Design review of the part built by this model. Coordinates are the model's own, in mm. A direction names the side the tool comes from. Round coordinates to 2 decimals unless told otherwise and drop trailing zeros. Order: outer loops, then holes, each group sorted by start corner. A loop starts at its lowest first (then second) coordinate and runs counter-clockwise, first axis right, second up.
Autodesk Inventor part; units mm, degrees
ref_plane "YZ Plane" through (0, 0, 0) normal (1, 0, 0) x (0, 1, 0)
ref_plane "XZ Plane" through (0, 0, 0) normal (0, 1, 0) x (-1, 0, 0)
ref_plane "XY Plane" through (0, 0, 0) normal (0, 0, 1) x (1, 0, 0)
sketch "Sketch1" plane through (0, 0, 0) normal (0, 0, 1) x (1, 0, 0)
  line L0 (19.05, -19.05) -> (-19.05, -19.05)
  line L1 (-19.05, -19.05) -> (-19.05, 19.05)
  line L2 (-19.05, 19.05) -> (19.05, 19.05)
  line L3 (19.05, 19.05) -> (19.05, -19.05)
  line L4 (19.05, -19.05) -> (-19.05, 19.05) construction
  line L5 (-19.05, -19.05) -> (19.05, 19.05) construction
  line L6 (-19.05, 19.05) -> (19.05, 19.05)
  line L7 (19.05, 19.05) -> (19.05, 44.45)
  line L8 (19.05, 44.45) -> (-19.05, 44.45)
  line L9 (-19.05, 44.45) -> (-19.05, 19.05)
  line L10 (0, 19.05) -> (0, 82.55)
  circle A0 centre (0, 82.55) radius 47.625
  circle A1 centre (0, 82.55) radius 28.575
  point P0 (0, 0)
  dimension "d0" = 38.1
  dimension "d1" = 38.1
  dimension "d2" = 25.4
  dimension "d3" = 63.5
  dimension "d4" = 95.25
  dimension "d5" = 57.15
extrude "Extrusion1" add sketch "Sketch1" along normal blind 3.175
sketch "Sketch2" plane through (0, 0, 3.175) normal (0, 0, 1) x (1, 0, 0)
  circle A0 centre (0, 82.55) radius 28.575 construction
  arc A1 (19.05, 38.901) -> (-19.05, 38.901) centre (0, 82.55) ccw construction
  line L0 (-19.05, 38.901) -> (-19.05, -19.05) construction
  line L1 (-19.05, -19.05) -> (19.05, -19.05) construction
  line L2 (19.05, -19.05) -> (19.05, 38.901) construction
  line L3 (-19.05, -19.05) -> (19.05, -19.05) construction
  line L4 (19.05, -19.05) -> (19.05, 19.05) construction
  line L5 (19.05, 19.05) -> (-19.05, 19.05) construction
  line L6 (-19.05, 19.05) -> (-19.05, -19.05) construction
  line L7 (15.875, -11.43) -> (-15.875, -11.43) construction
  line L8 (-15.875, -11.43) -> (-15.875, 11.43) construction
  line L9 (-15.875, 11.43) -> (15.875, 11.43) construction
  line L10 (15.875, 11.43) -> (15.875, -11.43) construction
  line L11 (15.875, -11.43) -> (-15.875, 11.43) construction
  line L12 (-15.875, -11.43) -> (15.875, 11.43) construction
  line L13 (11.43, -15.875) -> (-11.43, -15.875) construction
  line L14 (-11.43, -15.875) -> (-11.43, 15.875) construction
  line L15 (-11.43, 15.875) -> (11.43, 15.875) construction
  line L16 (11.43, 15.875) -> (11.43, -15.875) construction
  line L17 (11.43, -15.875) -> (-11.43, 15.875) construction
  line L18 (-11.43, -15.875) -> (11.43, 15.875) construction
  line L19 (0, -8.4414) -> (8.4414, 0) construction
  line L20 (8.4414, 0) -> (0, 8.4414) construction
  line L21 (0, 8.4414) -> (-8.4414, 0) construction
  line L22 (-8.4414, 0) -> (0, -8.4414) construction
  line L23 (-5.969, -5.969) -> (5.969, 5.969) construction
  line L24 (5.969, -5.969) -> (-5.969, 5.969) construction
  line L25 (-8.4414, -8.4414) -> (8.4414, -8.4414) construction
  line L26 (8.4414, -8.4414) -> (8.4414, 8.4414) construction
  line L27 (8.4414, 8.4414) -> (-8.4414, 8.4414) construction
  line L28 (-8.4414, 8.4414) -> (-8.4414, -8.4414) construction
  line L29 (-8.4414, -8.4414) -> (8.4414, 8.4414) construction
  line L30 (8.4414, -8.4414) -> (-8.4414, 8.4414) construction
  point P0 (0, 0)
  point P1 (0, 8.4414)
  point P2 (8.4414, 0)
  point P3 (-15.875, 0)
  point P4 (15.875, 0)
  dimension "d8" = 38.1
  dimension "d9" = 38.1
  dimension "d10" = 31.75
  dimension "d11" = 22.86
  dimension "d12" = 22.86
  dimension "d13" = 31.75
  dimension "d14" = 11.938
  dimension "d15" = 11.938
  dimension "d16" = 16.8829
  dimension "d17" = 16.8829
  dimension "d18" = 4.445
  dimension "d19" = 7.4336
  dimension "d20" = 5.969
  dimension "d21" = 5.969
  dimension "d22" = 4.445
  dimension "d23" = 7.4336
  dimension "d24" = 9.906
  dimension "d25" = 9.906
  dimension "d26" = 21.844
  dimension "d27" = 21.844
  dimension "d28" = 3.175
  dimension "d29" = 27.4914
hole "Hole1" at (-15.875, 11.43, 3.175) at (-15.875, 0, 3.175) at (-15.875, -11.43, 3.175) at (15.875, -11.43, 3.175) at (15.875, 0, 3.175) at (15.875, 11.43, 3.175) at (0, 8.4414, 3.175) at (0, -8.4414, 3.175) at (8.4414, 0, 3.175) at (-8.4414, 0, 3.175) direction (0, 0, -1) diameter 3.7973 end through all
properties part number "goniometer_stage_top_v1" material "Stainless Steel AISI 304"
1) Take a section at A-A on y = 0. Give the boundary of the cut face in (x, z) (3 decimals).
Results:
outline: (-19.05, 0) - (-17.774, 0) - (-17.774, 3.175) - (-19.05, 3.175) - close; (-13.976, 0) - (-10.34, 0) - (-10.34, 3.175) - (-13.976, 3.175) - close; (-6.543, 0) - (6.543, 0) - (6.543, 3.175) - (-6.543, 3.175) - close; (10.34, 0) - (13.976, 0) - (13.976, 3.175) - (10.34, 3.175) - close; (17.774, 0) - (19.05, 0) - (19.05, 3.175) - (17.774, 3.175) - close
2) For faces 1 (the face through (-17.476, 10.409, 1.565)), 2 (the face through (-19.05, 10, 2)), list the 3-axis set-ups (+Z, -Z, +X, -X, +Y, -Y) from which the entire face can be reached by the end or side of a thin tool; tool diameter is ignored.
Results:
face 1: +Z, -Z
face 2: +Z, -Z, -X, -Y
3) Take a section at B-B on x = 0. Give the boundary of the cut face in (y, z) (3 decimals), plus the area to 3 significant figures.
Results:
outline: (-19.05, 0) - (-10.34, 0) - (-10.34, 3.175) - (-19.05, 3.175) - close; (-6.543, 0) - (6.543, 0) - (6.543, 3.175) - (-6.543, 3.175) - close; (10.34, 0) - (53.975, 0) - (53.975, 3.175) - (10.34, 3.175) - close; (111.125, 0) - (130.175, 0) - (130.175, 3.175) - (111.125, 3.175) - close
area: 268 mm2
4) Take a section at C-C on y = 94. Give the boundary of the cut face in (x, z) (3 decimals).
Results:
outline: (-46.228, 0) - (-26.181, 0) - (-26.181, 3.175) - (-46.228, 3.175) - close; (26.181, 0) - (46.228, 0) - (46.228, 3.175) - (26.181, 3.175) - close
5) The part is to be moulded in two halves that separate along Y. For faces 3 (the face through (0, -19.05, 2)), 4 (the face through (6.56, 0.25, 1.57)), 5 (the face through (19.05, 10, 2)), say which applies: released by +Y, released by -Y, zero draft, split by the parting line, or undercut.
Results:
face 3: released by -Y
face 4: undercut
face 5: zero draft
6) Take a section at D-D on z = 1.2. State how many separate pieces and enclosed holes the cut face has, plus the area to 3 significant figures.
Results:
separate pieces: 1
enclosed holes: 11
area: 6,550 mm2
7) Clearance check with flat-ended pins moving along their axes: P1, Ø6, axis at x = -15.875, y = 11.43, coming from the -Z side; P2, Ø3.5, axis at x = 8.44, y = 0, coming from the -Z side; P3, Ø1, axis at y = 11, z = 1.5, coming from the -X side. State where each tip first meets the part, or that it passes through.
Results:
P1: stops at z = 0
P2: passes through
P3: stops at x = -19.05
8) To check wall thickness, follow line 1 along Y through (x, z) = (0, 1.15) (3 decimals); line 2 along X through (y, z) = (0, 1.5); line 3 along X through (y, z) = (11.43, 2.45). State the ranges of each line that lie inside material, in increasing order.
Results:
line 1: y = -19.05 to -10.34, -6.543 to 6.543, 10.34 to 53.975, 111.125 to 130.175
line 2: x = -19.05 to -17.77, -13.98 to -10.34, -6.54 to 6.54, 10.34 to 13.98, 17.77 to 19.05
line 3: x = -19.05 to -17.77, -13.98 to 13.98, 17.77 to 19.05
